Work out the finished part from the listing and answer in its coordinate system (mm). Coordinates: 2 decimals unless noted, no trailing zeros. Write each loop counter-clockwise with the first axis right and the second up, starting at its lowest first coordinate (ties: lowest second). Pieces come first, ordered by that corner, then holes. Notation, with made-up numbers: (11.25, 10) - (47.25, 10) arc R26 ccw to (47.25, 30) - close; hole circle Ø5 at (45.5, 39). An arc over 180 degrees is marked (long way). Use one line per item in the form item = value. Start each with the question number.
Item 1: Determine the mould class of faces 1 (the cylindrical face through (0.86, -3.131, 46.926)), 2 (the cylindrical face through (-6.435, -3.131, 2.026)), 3 (the flat face through (-25.4, -3, 26)), 4 (the cylindrical face through (0.559, -3.131, 76.194)) for opening direction Z: released by +Z, released by -Z, zero draft, split by the parting line, or undercut.
Item 2: Given pin 1 (2 mm diameter, centred on x = 1.5, y = -4.5, fed in from -Z); pin 2 (7 mm diameter, centred on x = 0, z = 50.8, fed in from -Y) (3 decimals), each flat-ended and moving along its own axis, determine where each tip first touches the part or whether it passes through.
Item 3: A cutting plane is placed at B-B (y = -3.25). Write down the section's boundary in (x, z).
Item 4: A cutting plane is placed at C-C (x = 12). Write down the section's boundary in (y, z), then the cut area to 3 significant figures.
Item 5: Consider probe 1 along Z at (x, y) = (0, -5); probe 2 along Z at (x, y) = (-19, -5.75); probe 3 along X at (y, z) = (-5.75, -11.5). Determine where each line is inside the solid, lowest interval first.
Item 6: A cutting plane is placed at A-A (x = 0). Write down the section's boundary in (y, z).
from build123d import *

# Parameters (mm, degrees)
F1_DEPTH = 6.35
F3_D     = 7.9375
F5_D     = 13.49248


with BuildPart() as f1:
    # F0 (on Front) → F1 (new body)
    with BuildSketch(Plane.XZ):
        with BuildLine():
            Line((-25.4, 50.8), (-25.4, 0))
            ThreePointArc((-25.4, 0), (0, -25.4), (25.4, 0))
            Line((25.4, 0), (25.4, 50.8))
            ThreePointArc((25.4, 50.8), (0, 76.2), (-25.4, 50.8))
        make_face()
    extrude(amount=F1_DEPTH)

    # F3 (through all)
    with Locations(Plane.XZ.offset(6.35)):
        with Locations((0, 50.8)):
            Hole(F3_D / 2)

    # F5 (through all)
    with Locations(Plane.XZ.offset(6.35)):
        with Locations((0, 0)):
            Hole(F5_D / 2)


solid = f1.part
Answer:
q1.face_1 = undercut
q1.face_2 = undercut
q1.face_3 = zero draft
q1.face_4 = released by +Z
q2.pin_1 = -25.4
q2.pin_2 = through
q3.outline = (-25.4, 0) arc R25.4 ccw to (25.4, 0) - (25.4, 50.8) arc R25.4 ccw to (-25.4, 50.8) - close; hole circle Ø13.49 at (0, 0); hole circle Ø7.94 at (0, 50.8)
q4.outline = (-6.35, -22.39) - (0, -22.39) - (0, 73.19) - (-6.35, 73.19) - close
q4.area = 607 mm²
q5.probe_1 = -25.4 to -6.75, 6.75 to 46.83, 54.77 to 76.2
q5.probe_2 = -16.86 to 67.66
q5.probe_3 = -22.65 to 22.65
q6.outline = (-6.35, -25.4) - (0, -25.4) - (0, -6.75) - (-6.35, -6.75) - close; (-6.35, 6.75) - (0, 6.75) - (0, 46.83) - (-6.35, 46.83) - close; (-6.35, 54.77) - (0, 54.77) - (0, 76.2) - (-6.35, 76.2) - close
